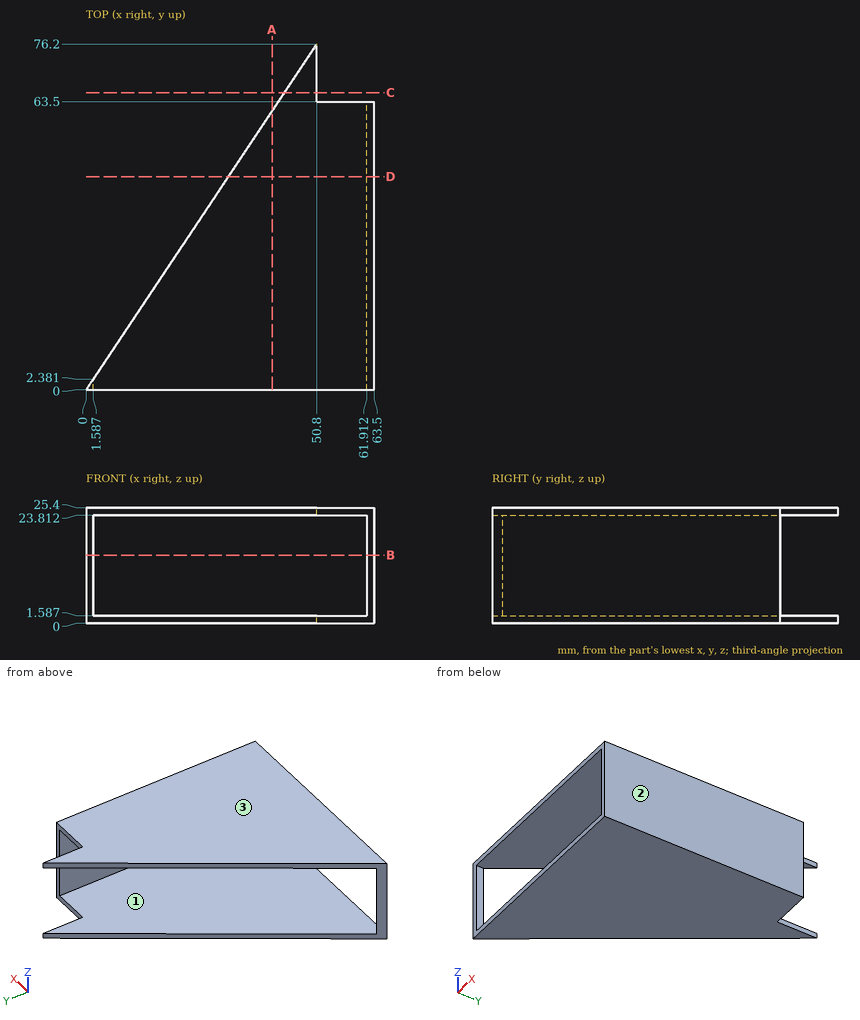
Source: three-view drawing plus pictorial views. Frame: mm from the lowest corner of the part. Give positions to 0.01 mm unless a question says otherwise; leave off trailing zeros. Order: outer loops, then holes, each group sorted by start corner. A loop starts at its lowest first (then second) coordinate and runs counter-clockwise, first axis right, second up. Notation, with made-up numbers: (49.5, -21) - (97.5, -21) arc R28 ccw to (97.5, -2) - close; hole circle Ø11 at (-36.5, 78). An arc over 180 degrees is marked (long way). Put each result on its own line as item: value.
Item 1: Draft query along Z for the marked faces 1, 2 and 3. Return one class per face: +Z half, -Z half, draft (parallel to the pull), parting line (faces both ways), or undercut.
Found:
face 1: undercut
face 2: draft
face 3: +Z half
Item 2: Section query B-B, the plane z = 15. Return loops of the section in (x, y), then the cut area to 3 significant figures.
Found:
outline: (0, 0) - (1.59, 0) - (1.59, 2.38) - close; (61.91, 0) - (63.5, 0) - (63.5, 63.5) - (61.91, 63.5) - close
area: 103 mm^2
Item 3: Section query A-A, the plane x = 41. Return loops of the section in (y, z).
Found:
outline: (0, 0) - (61.5, 0) - (61.5, 1.59) - (0, 1.59) - close; (0, 23.81) - (61.5, 23.81) - (61.5, 25.4) - (0, 25.4) - close
Item 4: Ray query, L1, parallel to Z at x = 15, y = 13.5; L2, parallel to X at y = 49.5, z = 9; L3, parallel to X at y = 34, z = 24 (1 decimal). Return the intervals inside material, ascending. Write a range as from..to.
Found:
L1: z = 0..1.59, 23.81..25.4
L2: x = 61.91..63.5
L3: x = 22.7..63.5
Item 5: Contact query for flat-ended pins moving along their axis: pin 1 (12 mm diameter, centred on y = 22, z = 5, fed in from -X) (1 decimal); pin 2 (10 mm diameter, centred on x = 57.5, z = 9.5, fed in from +Y); pin 3 (8 mm diameter, centred on x = 47, z = 16, fed in from +Y); pin 4 (1.3 mm diameter, centred on y = 70, z = 0.5, fed in from +X). Output: stop coordinate, or through.
Found:
pin 1: stops at x = 11.4
pin 2: stops at y = 63.5
pin 3: passes through
pin 4: stops at x = 50.8
Item 6: Section query D-D, the plane y = 47. Return loops of the section in (x, z).
Found:
outline: (31.33, 0) - (63.5, 0) - (63.5, 25.4) - (31.33, 25.4) - (31.33, 23.81) - (61.91, 23.81) - (61.91, 1.59) - (31.33, 1.59) - close
Item 7: Section query C-C, the plane y = 65.5. Return loops of the section in (x, z).
Found:
outline: (43.67, 0) - (50.8, 0) - (50.8, 1.59) - (43.67, 1.59) - close; (43.67, 23.81) - (50.8, 23.81) - (50.8, 25.4) - (43.67, 25.4) - close
